Read the model definition and answer for the solid it produces. Units are mm, in the model's axes. A direction names the side the tool comes from. Give positions to 0.01 mm unless a question says otherwise; leave off trailing zeros. Write each loop counter-clockwise with the first axis right and the second up, starting at its lowest first coordinate (ties: lowest second). Pieces come first, ordered by that corner, then holes. Notation, with made-up numbers: M 34,-22.75 L 57,-22.75 A20 cw 57,-2.75 Z; hole C 82.25,-15.5 d5. An arc over 180 degrees is marked long. Put each result on its own line as item: value.
from build123d import *

# Parameters (mm, degrees)
EXTRUDE_1_DEPTH     = 180
SKETCH_2_W          = 180
SKETCH_2_H          = 17.5
CUT_EXTRUDE_1_DEPTH = 45
SKETCH_3_W          = 180
SKETCH_3_H          = 37
CUT_EXTRUDE_2_DEPTH = 25
SKETCH_4_R          = 5
CUT_EXTRUDE_3_DEPTH = 10


with BuildPart() as part:
    # Эскиз1 → Вытянуть-Тонкостенный1 (new body)
    with BuildSketch(Plane(origin=(0, 0, 0), x_dir=(0, 0, -1), z_dir=(1, 0, 0))):
        with BuildLine():
            Line((-2, 55), (-2, 1))
            ThreePointArc((-2, 1), (-1.121320344, -1.121320344), (1, -2))
            Line((1, -2), (35, -2))
            ThreePointArc((35, -2), (37.121320344, -1.121320344), (38, 1))
            Line((38, 1), (38, 55))
            ThreePointArc((38, 55), (37.121320344, 57.121320344), (35, 58))
            Line((35, 58), (1, 58))
            ThreePointArc((1, 58), (-1.121320344, 57.121320344), (-2, 55))
        make_face()
        with BuildLine():
            Line((0, 55), (0, 1))
            ThreePointArc((0, 1), (0.292893219, 0.292893219), (1, 0))
            Line((1, 0), (35, 0))
            ThreePointArc((35, 0), (35.707106781, 0.292893219), (36, 1))
            Line((36, 1), (36, 55))
            ThreePointArc((36, 55), (35.707106781, 55.707106781), (35, 56))
            Line((35, 56), (1, 56))
            ThreePointArc((1, 56), (0.292893219, 55.707106781), (0, 55))
        make_face(mode=Mode.SUBTRACT)
    extrude(amount=EXTRUDE_1_DEPTH)

    # Эскиз2 → Вырез-Вытянуть1 (cut)
    with BuildSketch(Plane.XZ.offset(2)):
        with Locations((90, -6.75)):
            Rectangle(SKETCH_2_W, SKETCH_2_H)
    extrude(amount=-CUT_EXTRUDE_1_DEPTH, mode=Mode.SUBTRACT)

    # Эскиз3 → Вырез-Вытянуть2 (cut)
    with BuildSketch(Plane(origin=(0, 58, 0), x_dir=(1, 0, 0), z_dir=(0, 1, 0))):
        with Locations((90, 16.5)):
            Rectangle(SKETCH_3_W, SKETCH_3_H)
    extrude(amount=-CUT_EXTRUDE_2_DEPTH, mode=Mode.SUBTRACT)

    # Эскиз4 → Вырез-Вытянуть3 (cut)
    with BuildSketch(Plane(origin=(0, 0, -38), x_dir=(-1, 0, 0), z_dir=(0, 0, -1))):
        with Locations((-25, 32)):
            Circle(SKETCH_4_R)
    extrude(amount=-CUT_EXTRUDE_3_DEPTH, mode=Mode.SUBTRACT)


solid = part.part
(1) Given pin 1 Ø8 at (x, z) = (22.5, -27) entering from +Y; pin 2 Ø2 at (x, y) = (125.5, 57) entering from +Z; pin 3 Ø13 at (x, y) = (25, 32) entering from -Z; pin 4 Ø8 at (x, y) = (71, 43.5) entering from +Z, each flat-ended and moving along its own axis, determine where each tip first touches the part or whether it passes through.
Result:
pin 1: stops at y = 0
pin 2: stops at z = -35
pin 3: stops at z = -38
pin 4: stops at z = -36
(2) For a pull along Y with two mould halves and no side action, classify faces 3 (the face through (180, 19, -37)), 4 (the face through (89, 28, -36)), 5 (the face through (88.74, -1.14, -37.1)) as +Y half, -Y half, draft (parallel to the pull), parting line (faces both ways), or undercut.
Result:
face 3: draft
face 4: undercut
face 5: -Y half
(3) Section B-B on y = 32 is taken. Determine the outline of the cut face in (x, z), and give its area (3 significant figures).
Result:
outline: M 0,-38 L 20,-38 L 20,-36 L 0,-36 Z; M 30,-38 L 180,-38 L 180,-36 L 30,-36 Z
area: 340 mm²
(4) Section D-D on z = -17.25 is taken. Determine the outline of the cut face in (x, y), and give its area (3 significant figures).
Result:
outline: M 0,-2 L 180,-2 L 180,0 L 0,0 Z
area: 360 mm²
(5) Section A-A on x = 25 is taken. Determine the outline of the cut face in (y, z).
Result:
outline: M -2,-35 A3 ccw 1,-38 L 27,-38 L 27,-36 L 1,-36 A1 cw 0,-35 L 0,-15.5 L -2,-15.5 Z; M 37,-38 L 55,-38 A3 ccw 58,-35 L 56,-35 A1 cw 55,-36 L 37,-36 Z
(6) Section C-C on y = 11 is taken. Determine the outline of the cut face in (x, z), and give its area (3 significant figures).
Result:
outline: M 0,-38 L 180,-38 L 180,-36 L 0,-36 Z
area: 360 mm²
(7) Straight lines are drawn through the part: line 1 along Z through (x, y) = (73, 10.5); line 2 along Y through (x, z) = (39, -29); line 3 along Y through (x, z) = (25, -37.3). For each, find the intervals that lie inside material, in ascending order. Write a range as from..to.
Result:
line 1: z = -38..-36
line 2: y = -2..0
line 3: y = -0.93..27, 37..56.93
(8) Which of the six approach directions +Z, -Z, +X, -X, +Y, -Y give full straight-line access (tool end or side, diameter ignored) to faces 1 (the face through (88.74, 57.1, -37.14)), 2 (the face through (89, 0, -25))?
Result:
face 1: -Z, +X, -X, +Y
face 2: +Z, +X, -X, +Y
